Can you work these out from the drawing? Everything is in mm from the part's minimum corner. Give positions to 0.01 mm unless a question says otherwise; leave off trailing zeros. Loops run counter-clockwise (first coordinate to the right, second up) from the corner with the lowest first, then second, coordinate; pieces in that order, holes last. Notation, with made-up numbers: (51, 87.25) -> (76, 87.25) arc R24 ccw to (76, 100.25) -> close; hole circle Ø3 at (86, 80.25). An arc over 180 degrees is marked (long way). Write item = value, one per line. Start each with the question number.
1) I want a section at D-D (y = 91). List the corners of the cut face in (x, z) for me (1 decimal).
2) I'm going to push flat-ended pins straight in: pin 1 Ø1 at (y, z) = (68, 4) entering from -X; pin 2 Ø7.5 at (x, y) = (50.8, 7.92) entering from -Z; pin 3 Ø8 at (y, z) = (59.5, 1.5) entering from +X. Where does each tip first touch, or does it pass through?
3) I want a section at C-C (z = 9). Count the separate pieces of the cut face and the enclosed holes in it, and give its area (3 significant figures).
4) If we mould it in two halves opening along X, with no side actions, what happens to the marked faces 1, 2 and 3? For each: +X half, -X half, draft (parallel to the pull), parting line (faces both ways), or undercut.
5) I want a section at B-B (x = 50.8). List the corners of the cut face in (y, z) for me (1 decimal).
6) I want a section at A-A (y = 50.8). List the corners of the cut face in (x, z) for me (1 decimal), and give its area (3 significant figures).
7) I need wall thicknesses on probe 1 along Y at (x, z) = (50.8, 8.25); probe 2 along Y at (x, z) = (10.5, 4) (1 decimal); probe 3 along Y at (x, z) = (17.5, 12.75) (1 decimal). Which ranges of each line are inside material? Lowest first, please. Write a range as from..to.
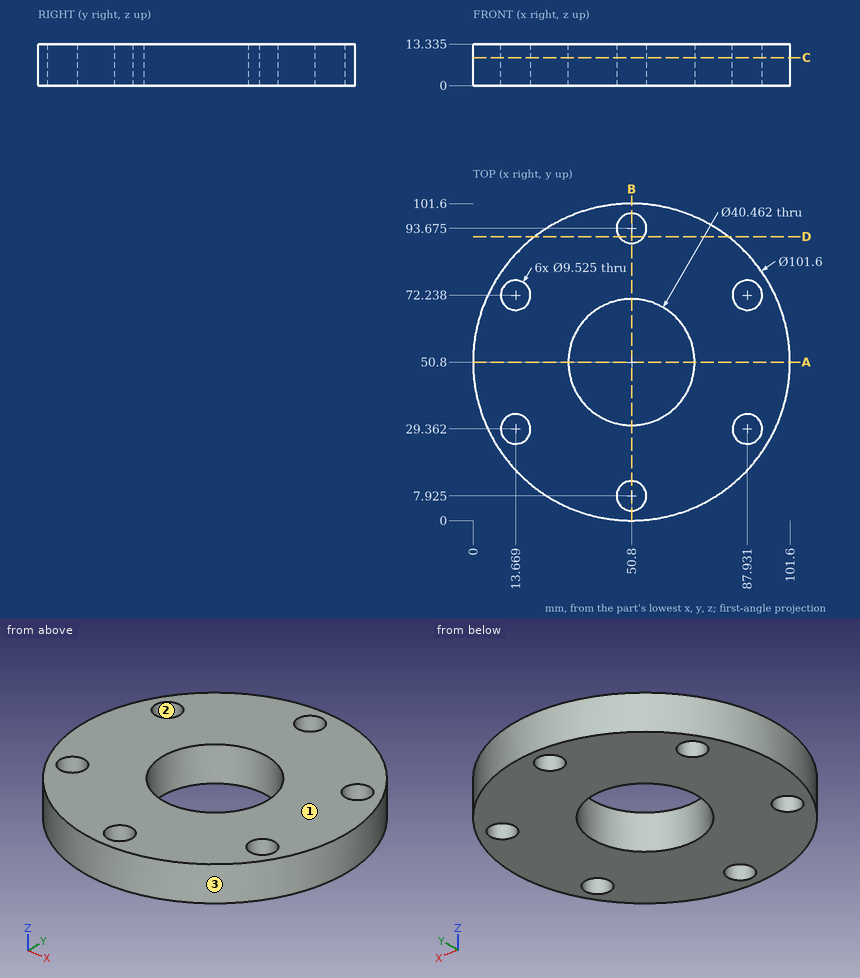
Answer list:
q1.outline = (19.7, 0) -> (46.9, 0) -> (46.9, 13.3) -> (19.7, 13.3) -> close; (54.7, 0) -> (81.9, 0) -> (81.9, 13.3) -> (54.7, 13.3) -> close
q2.pin_1 = 2.82
q2.pin_2 = through
q2.pin_3 = 101.38
q3.separate_pieces = 1
q3.enclosed_holes = 7
q3.area = 6,390 mm^2
q4.face_1 = draft
q4.face_2 = undercut
q4.face_3 = parting line
q5.outline = (0, 0) -> (3.2, 0) -> (3.2, 13.3) -> (0, 13.3) -> close; (12.7, 0) -> (30.6, 0) -> (30.6, 13.3) -> (12.7, 13.3) -> close; (71, 0) -> (88.9, 0) -> (88.9, 13.3) -> (71, 13.3) -> close; (98.4, 0) -> (101.6, 0) -> (101.6, 13.3) -> (98.4, 13.3) -> close
q6.outline = (0, 0) -> (30.6, 0) -> (30.6, 13.3) -> (0, 13.3) -> close; (71, 0) -> (101.6, 0) -> (101.6, 13.3) -> (71, 13.3) -> close
q6.area = 815 mm^2
q7.probe_1 = 0..3.16, 12.69..30.57, 71.03..88.91, 98.44..101.6
q7.probe_2 = 19.9..25.8, 32.9..68.7, 75.8..81.7
q7.probe_3 = 12.4..26.5, 32.2..69.4, 75.1..89.2
